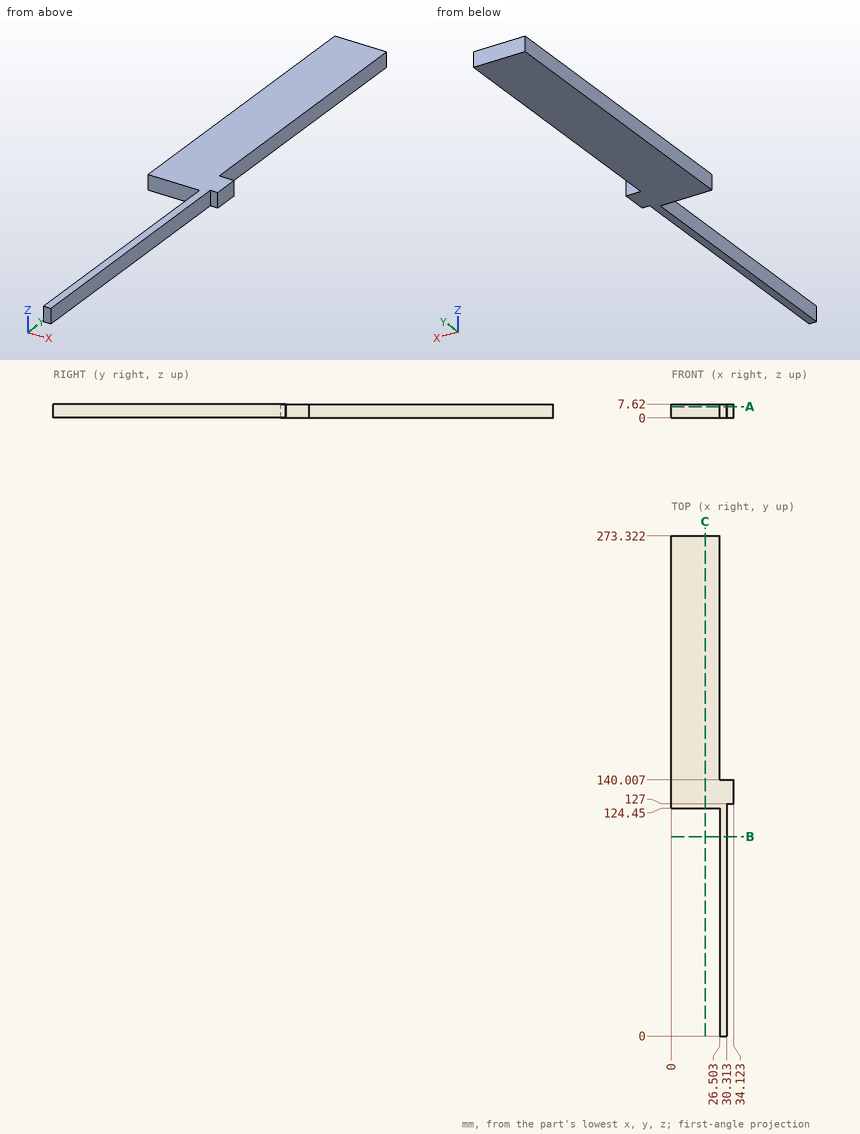
Input: dimensioned drawing with shaded views. Units: mm. Origin: part minimum x, y, z. Round coordinates to 2 decimals unless told otherwise and drop trailing zeros. Write each loop counter-clockwise with the first axis right and the second up, starting at its lowest first coordinate (ties: lowest second). Pieces come first, ordered by that corner, then holes. Notation, with made-up numbers: (63, 19) - (113, 19) arc R12 cw to (113, 34) - close; hole circle Ø10 at (36.25, -6). An arc over 180 degrees is marked (long way). Write item = value, one per line.
(1) Contact query for flat-ended pins moving along their axis: pin 1 Ø4 at (x, y) = (25, 217) entering from -Z; pin 2 Ø1 at (y, z) = (215.5, 3.5) entering from +X; pin 3 Ø1.9 at (x, z) = (32, 4) entering from -Y; pin 4 Ø2.5 at (x, z) = (11, 5) entering from -Y. Output: stop coordinate, or through.
Geometry check:
pin_1 = 0
pin_2 = 26.5
pin_3 = 127
pin_4 = 124.45
(2) Section query C-C on x = 18.5. Output: boundary loops of the cut face in (y, z), then the cut area to 3 significant figures.
Geometry check:
outline = (124.45, 0) - (273.32, 0) - (273.32, 7.62) - (124.45, 7.62) - close
area = 1,130 mm^2
(3) Section query A-A on z = 6.25. Output: boundary loops of the cut face in (x, y), then the cut area to 3 significant figures.
Geometry check:
outline = (0, 124.45) - (26.5, 124.45) - (26.5, 0) - (30.31, 0) - (30.31, 127) - (34.12, 127) - (34.12, 140.01) - (26.5, 140.01) - (26.5, 273.32) - (0, 273.32) - close
area = 4,530 mm^2
(4) Material intervals for probe 1 along X at (y, z) = (191, 4.75); probe 2 along Y at (x, z) = (27.5, 1); probe 3 along Y at (x, z) = (24, 6), sorted ascending.
Geometry check:
probe_1 = 0 to 26.5
probe_2 = 0 to 140.01
probe_3 = 124.45 to 273.32
(5) Section query B-B on y = 109. Output: boundary loops of the cut face in (x, z).
Geometry check:
outline = (26.5, 0) - (30.31, 0) - (30.31, 7.62) - (26.5, 7.62) - close
